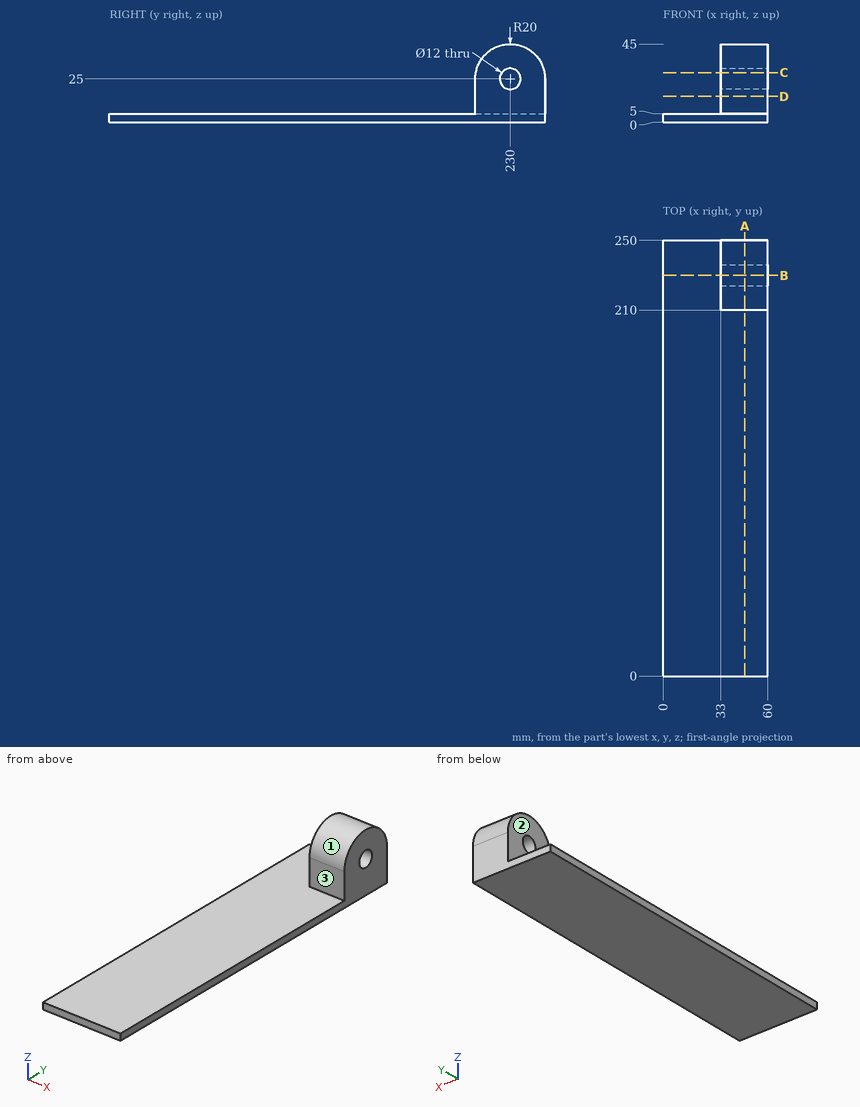
Can you work these out from the drawing? Everything is in mm from the part's minimum corner. A direction names the side the tool comes from. Round coordinates to 2 decimals unless told otherwise and drop trailing zeros. Loops run counter-clockwise (first coordinate to the right, second up) from the corner with the lowest first, then second, coordinate; pieces in that order, holes last. Notation, with made-up numbers: (-6, -8.5) -> (-2, -8.5) arc R17 ccw to (-2, 21.5) -> close; hole circle Ø3 at (-23.75, 63). An arc over 180 degrees is marked (long way). Answer in a Markdown table with one row per item.
Item 1: Suppose I cut it at D-D, the plane z = 15. List the corners of the cut face in (x, y) for me, plus the area to 3 significant figures.
Answer block:
| item | result |
|---|---|
| outline | (33, 210) -> (60, 210) -> (60, 250) -> (33, 250) -> close |
| area | 1,080 mm² |
Item 2: Suppose I cut it at B-B, the plane y = 230. List the corners of the cut face in (x, z) for me.
Answer block:
| item | result |
|---|---|
| outline | (0, 0) -> (60, 0) -> (60, 19) -> (33, 19) -> (33, 5) -> (0, 5) -> close; (33, 31) -> (60, 31) -> (60, 45) -> (33, 45) -> close |
Item 3: On a 3-axis mill with a long thin cutter (end or side, diameter ignored), from which of +Z, -Z, +X, -X, +Y, -Y can I reach the whole of each face in a straight line? I mean the marked faces 1, 2 and 3. Say none if no direction works.
Answer block:
| item | result |
|---|---|
| face 1 | +Z, +X, -X |
| face 2 | +Z, -X, +Y, -Y |
| face 3 | +Z, +X, -X, -Y |
Item 4: Will these pins go through, and if not, where does the flat tip stop? P1, Ø7, axis at y = 230, z = 25, coming from the -X side; P2, Ø3, axis at x = 36, z = 28, coming from the +Y side; P3, Ø3, axis at x = 45, z = 33.5, coming from the -Y side (3 decimals).
Answer block:
| item | result |
|---|---|
| P1 | through |
| P2 | y = 249.94 |
| P3 | y = 211.265 |
Item 5: If I drill on probe 1 along Y at (x, z) = (40, 25); probe 2 along Z at (x, y) = (53.5, 75.5); probe 3 along X at (y, z) = (217, 13), over which ranges is the centre line in solid material (lowest first)?
Answer block:
| item | result |
|---|---|
| probe 1 | 210 to 224, 236 to 250 |
| probe 2 | 0 to 5 |
| probe 3 | 33 to 60 |
Item 6: Suppose I cut it at A-A, the plane x = 47. List the corners of the cut face in (y, z) for me, plus the area to 3 significant figures.
Answer block:
| item | result |
|---|---|
| outline | (0, 0) -> (250, 0) -> (250, 25) arc R20 ccw to (210, 25) -> (210, 5) -> (0, 5) -> close; hole circle Ø12 at (230, 25) |
| area | 2,570 mm² |
Item 7: Suppose I cut it at C-C, the plane z = 28.5. List the corners of the cut face in (x, y) for me.
Answer block:
| item | result |
|---|---|
| outline | (33, 210.31) -> (60, 210.31) -> (60, 225.13) -> (33, 225.13) -> close; (33, 234.87) -> (60, 234.87) -> (60, 249.69) -> (33, 249.69) -> close |
